from build123d import *

# Parameters (mm, degrees)
F1_DEPTH = 6.35
F2_W     = 3.175
F2_H     = 3.175
F2_H_2   = 101.6
F2_W_2   = 88.9
F2_W_3   = 32.385
F2_W_4   = 22.225
F3_DEPTH = 20.6375
F4_W     = 38.1
F4_H     = 20.6375
F5_DEPTH = 3.175


with BuildPart() as f1:
    # F0 (on Top) → F1 (new body)
    with BuildSketch(Plane.XY):
        Polygon((59.69, 52.148615), (-35.56, 52.148615), (-35.56, -55.801385), (0, -55.801385), (0, 33.098615), (34.29, 33.098615), (34.29, -55.801385), (59.69, -55.801385), align=None)
    extrude(amount=F1_DEPTH)

    # F2 (on face) → F3 (join)
    with BuildSketch(Plane.XY.offset(6.35)):
        with Locations((-33.9725, -54.213885)):
            Rectangle(F2_W, F2_H)
        with Locations((-33.9725, -1.826385)):
            Rectangle(F2_W, F2_H_2)
        with Locations((-33.9725, 50.561115)):
            Rectangle(F2_W, F2_H)
        with Locations((12.065, 50.561115)):
            Rectangle(F2_W_2, F2_H)
        with Locations((58.1025, -1.826385)):
            Rectangle(F2_W, F2_H_2)
        with Locations((58.1025, 50.561115)):
            Rectangle(F2_W, F2_H)
        with Locations((58.1025, -54.213885)):
            Rectangle(F2_W, F2_H)
        with Locations((-16.1925, -54.213885)):
            Rectangle(F2_W_3, F2_H)
        with Locations((45.4025, -54.213885)):
            Rectangle(F2_W_4, F2_H)
    extrude(amount=F3_DEPTH)

    # F4 (on face) → F5 (cut)
    with BuildSketch(Plane.YZ.offset(59.69)):
        with Locations((7.698615, 16.66875)):
            Rectangle(F4_W, F4_H)
    extrude(amount=-F5_DEPTH, mode=Mode.SUBTRACT)


solid = f1.part
Check sheet for the modelled part. Datum: model origin and axes. Units: mm. A direction names the side the tool comes from. Coordinates: 2 decimals unless noted, no trailing zeros. Loops run counter-clockwise (first coordinate to the right, second up) from the corner with the lowest first, then second, coordinate; pieces in that order, holes last. Notation, with made-up numbers: (-7, -5.75) -> (33, -5.75) arc R23 ccw to (33, 24.25) -> close; hole circle Ø4 at (81.25, -15). An arc over 180 degrees is marked (long way). Write item = value, one per line. Start each with the question number.
1. Depth check by flat-ended pin: P1, Ø5, axis at y = 14, z = 11, coming from the +X side (3 decimals); P2, Ø10.5, axis at x = 17, z = 18.5, coming from the -Y side; P3, Ø5, axis at x = 24.5, z = 2.5, coming from the -Y side. Enter the tip coordinate at first touch or a pass-through.
2. Section check C-C on x = -17.5. Record the cut outline in (y, z), then the cut area to 3 significant figures.
3. Tool access check on faces 5 (the flat face through (-10, 11, 0)), 6 (the flat face through (13, 52.149, 13)), 7 (the flat face through (58, -11.351, 17)), 8 (the flat face through (56.515, -32, 17)), 9 (the flat face through (0, -18, 5)). Record the directions out of +Z, -Z, +X, -X, +Y, -Y that give a thin tool (end or side, any length) a straight path to the whole face; none if there is none.
4. Draft check along X on faces 1 (the flat face through (-35.56, -1, 13)), 2 (the flat face through (58, 26.749, 17)), 3 (the flat face through (56.515, 38, 17)), 4 (the flat face through (59.69, -15, 13)). Enter one of: released by +X, released by -X, zero draft, split by the parting line, or undercut.
5. Section check B-B on z = 25. Record the cut outline in (x, y) (3 decimals), then the cut area to 3 significant figures.
6. Material ranges on line 1 (Y direction, x = 52, z = 11); line 2 (X direction, y = -33.5, z = 12.5) (3 decimals); line 3 (X direction, y = -25, z = 3.75), recorded low to high.
Responses:
q1.P1 = -32.385
q1.P2 = 48.97
q1.P3 = 33.1
q2.outline = (-55.8, 0) -> (52.15, 0) -> (52.15, 26.99) -> (48.97, 26.99) -> (48.97, 6.35) -> (-52.63, 6.35) -> (-52.63, 26.99) -> (-55.8, 26.99) -> close
q2.area = 817 mm2
q3.face_5 = -Z, +X, -X, +Y, -Y
q3.face_6 = +Z, -Z, +X, -X, +Y
q3.face_7 = +Z, +X
q3.face_8 = +Z
q3.face_9 = +Z, -Z, -Y
q4.face_1 = released by -X
q4.face_2 = zero draft
q4.face_3 = undercut
q4.face_4 = released by +X
q5.outline = (-35.56, -55.801) -> (0, -55.801) -> (0, -52.626) -> (-32.385, -52.626) -> (-32.385, 48.974) -> (56.515, 48.974) -> (56.515, 26.749) -> (59.69, 26.749) -> (59.69, 52.149) -> (-35.56, 52.149) -> close; (34.29, -55.801) -> (59.69, -55.801) -> (59.69, -11.351) -> (56.515, -11.351) -> (56.515, -52.626) -> (34.29, -52.626) -> close
q5.area = 1,020 mm2
q6.line_1 = -55.8 to -52.63, 48.97 to 52.15
q6.line_2 = -35.56 to -32.385, 56.515 to 59.69
q6.line_3 = -35.56 to 0, 34.29 to 59.69
